Build history of the part. All positions in model axes, mm. Give positions to 0.01 mm unless a question says otherwise; leave off trailing zeros. Loops run counter-clockwise (first coordinate to the right, second up) from the corner with the lowest first, then second, coordinate; pieces in that order, holes last.
1) Wall check: line 1 (Z direction, x = -14, y = 0.65); line 2 (X direction, y = 1.5, z = 0); line 3 (Z direction, x = 12, y = 1). Give the ranges that are in metal, low to high.
2) Two-plate mould, pull along Y, no slides. Class faces 1 (the flat face through (0, 1, 6)), 2 (the flat face through (0, 0, -25)), 3 (the flat face through (0, 2, -25)): +Y half, -Y half, draft (parallel to the pull), parting line (faces both ways), or undercut.
3) Band-saw the part on B-B on y = 1.35. List the corners of the cut face in (x, z).
4) Band-saw the part on A-A on x = 15. List the corners of the cut face in (y, z).
```python
from build123d import *

# Parameters (mm, degrees)
EXTRUDE_1_DEPTH = 2


with BuildPart() as part:
    # 草图1 → 凸台-拉伸1 (new body)
    with BuildSketch(Plane(origin=(0, 0, 0), x_dir=(1, 0, 0), z_dir=(0, 1, 0))):
        with BuildLine():
            Line((-11.75, 0), (0, 0))
            Line((0, 0), (0, 30))
            Line((0, 30), (-11.75, 30))
            ThreePointArc((-11.75, 30), (-12.409009742, 28.409009742), (-14, 27.75))
            Line((-14, 27.75), (-14, 2.25))
            ThreePointArc((-14, 2.25), (-12.409009742, 1.590990258), (-11.75, 0))
        make_face()
        with BuildLine():
            Line((0, 30), (0, 0))
            Line((0, 0), (11.75, 0))
            ThreePointArc((11.75, 0), (12.409009742, 1.590990258), (14, 2.25))
            Line((14, 2.25), (14, 27.75))
            ThreePointArc((14, 27.75), (12.409009742, 28.409009742), (11.75, 30))
            Line((11.75, 30), (0, 30))
        make_face()
        with BuildLine():
            Line((11.75, 0), (0, 0))
            Line((0, 0), (-11.75, 0))
            ThreePointArc((-11.75, 0), (-15.590990258, -1.590990258), (-14, 2.25))
            Line((-14, 2.25), (-14, 27.75))
            ThreePointArc((-14, 27.75), (-16.25, 30), (-14, 32.25))
            Line((-14, 32.25), (-14, 46.75))
            ThreePointArc((-14, 46.75), (-15.75, 48.5), (-14, 50.25))
            Line((-14, 50.25), (-14, 56))
            Line((-14, 56), (-20, 56))
            Line((-20, 56), (-20, -3))
            ThreePointArc((-20, -3), (-19.121320344, -5.121320344), (-17, -6))
            Line((-17, -6), (17, -6))
            ThreePointArc((17, -6), (19.121320344, -5.121320344), (20, -3))
            Line((20, -3), (20, 56))
            Line((20, 56), (14, 56))
            Line((14, 56), (14, 50.25))
            ThreePointArc((14, 50.25), (15.237436867, 49.737436867), (15.75, 48.5))
            ThreePointArc((15.75, 48.5), (15.237436867, 47.262563133), (14, 46.75))
            Line((14, 46.75), (14, 32.25))
            ThreePointArc((14, 32.25), (15.590990258, 31.590990258), (16.25, 30))
            ThreePointArc((16.25, 30), (15.590990258, 28.409009742), (14, 27.75))
            Line((14, 27.75), (14, 2.25))
            ThreePointArc((14, 2.25), (15.590990258, 1.590990258), (16.25, 0))
            ThreePointArc((16.25, 0), (14, -2.25), (11.75, 0))
        make_face()
        with BuildLine():
            Line((-11.75, 30), (0, 30))
            Line((0, 30), (11.75, 30))
            ThreePointArc((11.75, 30), (12.409009742, 31.590990258), (14, 32.25))
            Line((14, 32.25), (14, 46.75))
            ThreePointArc((14, 46.75), (12.25, 48.5), (14, 50.25))
            Line((14, 50.25), (14, 56))
            Line((14, 56), (-14, 56))
            Line((-14, 56), (-14, 50.25))
            ThreePointArc((-14, 50.25), (-12.762563133, 49.737436867), (-12.25, 48.5))
            ThreePointArc((-12.25, 48.5), (-12.762563133, 47.262563133), (-14, 46.75))
            Line((-14, 46.75), (-14, 32.25))
            ThreePointArc((-14, 32.25), (-12.409009742, 31.590990258), (-11.75, 30))
        make_face()
    extrude(amount=EXTRUDE_1_DEPTH)


solid = part.part
```
Findings below:
1. line 1: z = -56 to -50.25, -46.75 to -32.25, -27.75 to -2.25, 2.25 to 6
1. line 2: x = -20 to -16.25, -11.75 to 11.75, 16.25 to 20
1. line 3: z = -56 to -31.03, -28.97 to -1.03, 1.03 to 6
2. face 1: draft
2. face 2: -Y half
2. face 3: +Y half
3. outline: (-20, -56) - (20, -56) - (20, 3) arc R3 ccw to (17, 6) - (-17, 6) arc R3 ccw to (-20, 3) - close; hole circle Ø4.5 at (-14, -30); hole circle Ø4.5 at (-14, 0); hole circle Ø3.5 at (-14, -48.5); hole circle Ø4.5 at (14, -30); hole circle Ø4.5 at (14, 0); hole circle Ø3.5 at (14, -48.5)
4. outline: (0, -56) - (2, -56) - (2, -49.94) - (0, -49.94) - close; (0, -47.06) - (2, -47.06) - (2, -32.02) - (0, -32.02) - close; (0, -27.98) - (2, -27.98) - (2, -2.02) - (0, -2.02) - close; (0, 2.02) - (2, 2.02) - (2, 6) - (0, 6) - close
